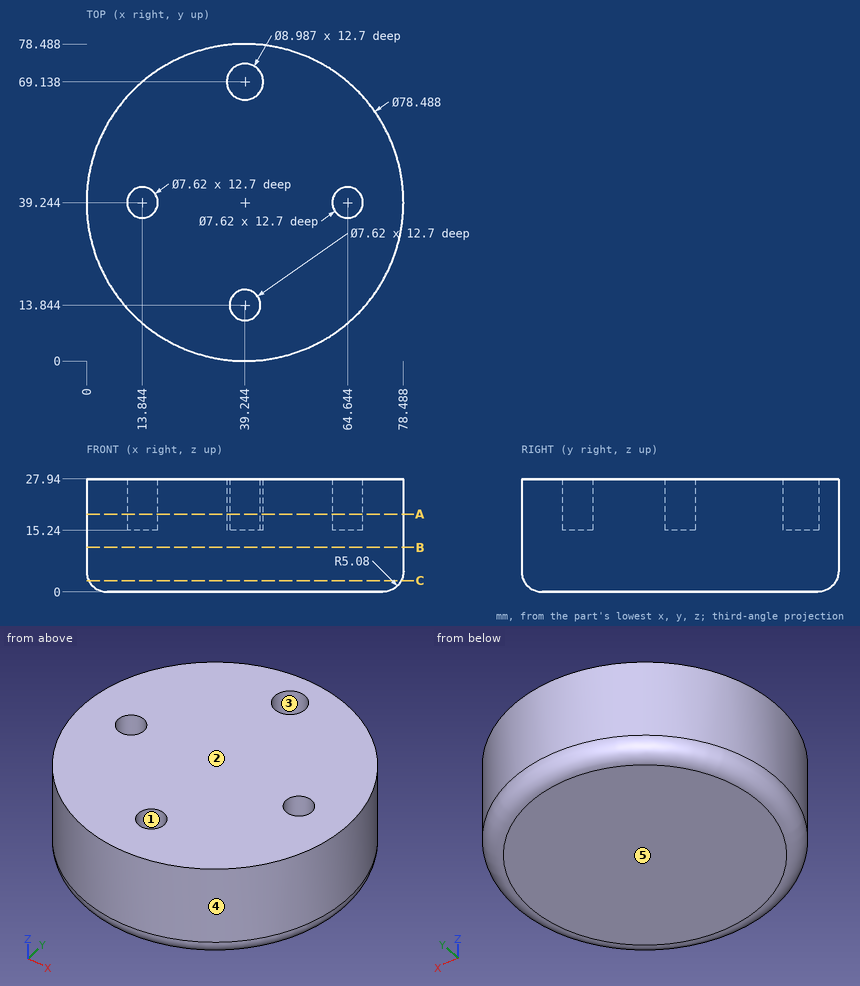
Can you work these out from the drawing? Everything is in mm from the part's minimum corner. A direction names the side the tool comes from. Coordinates: 2 decimals unless noted, no trailing zeros. Loops run counter-clockwise (first coordinate to the right, second up) from the corner with the lowest first, then second, coordinate; pieces in that order, holes last. Notation, with made-up numbers: M 63,43.25 L 103,43.25 A24 ccw 103,74.25 Z; hole C -35,-8.5 d4. An arc over 180 degrees is marked long. Put each result on its own line as item: value. Start each with the question number.
(1) Suppose I cut it at B-B on z = 11. Please give me the cut outline in (x, y) (1 decimal), then the cut area to 3 significant figures.
(2) I need wall thicknesses on line 1 (Y direction, x = 66, z = 21.75) (1 decimal); line 2 (X direction, y = 55, z = 22.25) (1 decimal); line 3 (Y direction, x = 24, z = 1.5). Which ranges of each line are inside material? Lowest first, please. Write a range as from..to.
(3) Suppose I cut it at C-C on z = 2.75. Please give me the cut outline in (x, y) (1 decimal).
(4) Thinking about a two-plate mould opening in Y: for the marked faces 3, 4 and 5, which applies, pulls with the +Y half, pulls with the -Y half, needs draft (parallel to the pull), parting line crosses it, or undercut?
(5) Suppose I cut it at A-A on z = 19.25. Please give me the cut outline in (x, y) (1 decimal), then the cut area to 3 significant figures.
(6) Will these pins go through, and if not, where does the flat tip stop? P1, Ø4, axis at x = 37.5, y = 12, coming from the +Z side; P2, Ø2, axis at x = 39, z = 6, coming from the -Y side; P3, Ø1.5, axis at x = 18.5, z = 7, coming from the +Y side; P4, Ø2.5, axis at x = 41, y = 70, coming from the +Z side.
(7) For the marked faces 1 and 2, which set-ups out of +Z, -Z, +X, -X, +Y, -Y let a thin tool reach every point of the face, with its end or its side?
Solutions:
1. outline: C 39.2,39.2 d78.5
1. area: 4,840 mm2
2. line 1: y = 10.5..35.7, 42.8..68
2. line 2: x = 3.3..75.2
2. line 3: y = 4.69..73.8
3. outline: C 39.2,39.2 d77.4
4. face 3: undercut
4. face 4: parting line crosses it
4. face 5: needs draft
5. outline: C 39.2,39.2 d78.5; hole C 13.8,39.2 d7.6; hole C 39.2,69.1 d9; hole C 39.2,13.8 d7.6; hole C 64.6,39.2 d7.6
5. area: 4,640 mm2
6. P1: stops at z = 27.94
6. P2: stops at y = 0
6. P3: stops at y = 73.01
6. P4: stops at z = 15.24
7. face 1: +Z
7. face 2: +Z, +X, -X, +Y, -Y
